from build123d import *

# Parameters (mm, degrees)
SKETCH2_R      = 6.4135
SKETCH2_R_2    = 4.826
EXTRUDE1_DEPTH = 38.1
EXTRUDE2_DEPTH = 25.4


with BuildPart() as part:
    # Sketch2 → Extrude1 (new body)
    with BuildSketch(Plane.XY.offset(-31.75)):
        with Locations((38.035581748, 37.774829094)):
            Circle(SKETCH2_R)
        with Locations((38.035581748, 37.774829094)):
            Circle(SKETCH2_R_2, mode=Mode.SUBTRACT)
    extrude(amount=EXTRUDE1_DEPTH)

    # Sketch3 → Extrude2 (add)
    with BuildSketch(Plane.XY.offset(6.35)):
        with BuildLine():
            Line((31.844396197, 36.10085068), (6.48762227, 10.917909932))
            ThreePointArc((6.48762227, 10.917909932), (9.011090735, 8.949315268), (10.962279904, 6.412364564))
            Line((10.962279904, 6.412364564), (36.319053831, 31.595305313))
            ThreePointArc((36.319053831, 31.595305313), (33.484980926, 33.255424883), (31.844396197, 36.10085068))
        make_face()
    extrude(amount=-EXTRUDE2_DEPTH)


solid = part.part
Check sheet for the modelled part. Datum: model origin and axes. Units: mm. Round coordinates to 2 decimals unless told otherwise and drop trailing zeros. Loops run counter-clockwise (first coordinate to the right, second up) from the corner with the lowest first, then second, coordinate; pieces in that order, holes last. Notation, with made-up numbers: M 42,63 L 95,63 A20 cw 95,91 Z; hole C -32,-31.75 d11. An arc over 180 degrees is marked long. One line per question, with ' | ' between items. Start each with the question number.
Item 1: Gauge pin test, flat ends, axial feed: pin 1 Ø12 at (y, z) = (19, -7) entering from -X; pin 2 Ø1 at (x, z) = (14, 0.5) entering from +Y; pin 3 Ø4 at (x, z) = (20.5, -4) entering from +Y. Record the tip position at first contact, or that the pin passes through.
Item 2: Section check A-A (y = 37). Record the boundary of the cut face in (x, z), and give its area (3 significant figures).
Item 3: Section check D-D (x = 32.5). Record the boundary of the cut face in (y, z).
Item 4: Section check C-C (z = -7.5). Record the boundary of the cut face in (x, y).
Item 5: Section check B-B (x = 37). Record the boundary of the cut face in (y, z).
Item 6: Scan lines: probe 1 along X at (y, z) = (37.5, -2); probe 2 along Z at (x, y) = (25.5, 21); probe 3 along X at (y, z) = (41.5, -24). Record each from-to range of solid material in increasing order.
Item 7: Release check for a two-part mould opening along X. For faces 1 (the face through (39, 43, -31.75)), 2 (the face through (19.344, 23.686, -6.172)), 3 (the face through (34.48, 41.04, -12.97)) record: released by +X, released by -X, zero draft, split by the parting line, or undercut.
Worked out:
1) pin 1: x = 8.58 | pin 2: y = 18.88 | pin 3: y = 26.82
2) outline: M 31.67,-31.75 L 33.27,-31.75 L 33.27,6.35 L 31.67,6.35 Z; M 42.8,-31.75 L 44.4,-31.75 L 44.4,6.35 L 42.8,6.35 Z | area: 122 mm^2
3) outline: M 27.8,-19.05 L 34.54,-19.05 L 34.54,-31.75 L 41.01,-31.75 L 41.01,6.35 L 27.8,6.35 Z
4) outline: M 6.49,10.92 A12.7 cw 10.96,6.41 L 36.32,31.6 A6.41 ccw long 31.84,36.1 Z; hole C 38.04,37.77 d9.65
5) outline: M 31.45,-31.75 L 33.06,-31.75 L 33.06,6.35 L 31.45,6.35 Z; M 42.49,-31.75 L 44.1,-31.75 L 44.1,6.35 L 42.49,6.35 Z
6) probe 1: 31.63 to 33.22, 42.85 to 44.44 | probe 2: -19.05 to 6.35 | probe 3: 32.81 to 34.97, 41.1 to 43.26
7) face 1: zero draft | face 2: released by -X | face 3: undercut
